Here's the drawing with two shaded views (mm, measured from the low corner). I have some questions. A direction names the side the tool comes from. Coordinates: 2 decimals unless noted, no trailing zeros. Loops run counter-clockwise (first coordinate to the right, second up) from the corner with the lowest first, then second, coordinate; pieces in that order, holes last.
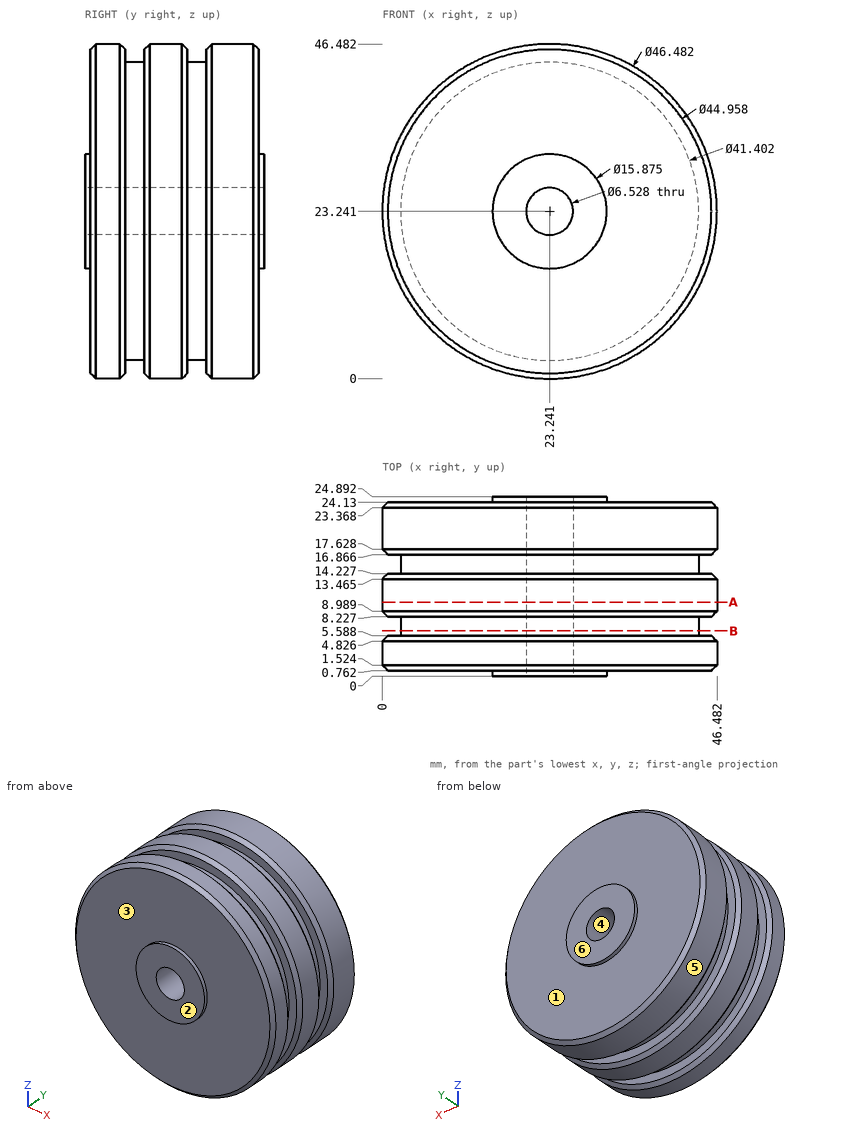
Q1. We'd pull the mould along Z, two halves only. Please class the marked faces 4, 5 and 6: pulls with the +Z half, pulls with the -Z half, needs draft (parallel to the pull), parting line crosses it, or undercut.
Q2. Suppose I cut it at B-B on y = 6.25. Write out the boundary of the cut face in (x, z).
Q3. For the marked faces 1, 2 and 3, which set-ups out of +Z, -Z, +X, -X, +Y, -Y let a thin tool reach every point of the face, with its end or its side?
Q4. Suppose I cut it at A-A on y = 10.25. Write out the boundary of the cut face in (x, z).
Q5. Please list where these lines run through material, in increasing order: probe 1 along Y at (x, z) = (18.5, 44) (1 decimal); probe 2 along Y at (x, z) = (33.5, 3) (1 decimal); probe 3 along Y at (x, z) = (14, 24.5).
Q6. Will these pins go through, and if not, where does the flat tip stop? P1, Ø4, axis at x = 8.5, z = 10.5, coming from the +Y side; P2, Ø6, axis at x = 39, y = 12, coming from the -Z side (1 decimal); P3, Ø10, axis at y = 7.5, z = 33.5, coming from the -X side.
Check values:
1. face 4: undercut
1. face 5: parting line crosses it
1. face 6: needs draft
2. outline: circle Ø41.4 at (23.24, 23.24); hole circle Ø6.53 at (23.24, 23.24)
3. face 1: +Y
3. face 2: +Z, -Z, +X, -X, -Y
3. face 3: -Y
4. outline: circle Ø46.48 at (23.24, 23.24); hole circle Ø6.53 at (23.24, 23.24)
5. probe 1: y = 0.8 to 5.6, 8.2 to 14.2, 16.9 to 24.1
5. probe 2: y = 1 to 5.4, 8.4 to 14, 17.1 to 23.9
5. probe 3: y = 0.76 to 24.13
6. P1: stops at y = 24.13
6. P2: stops at z = 3.8
6. P3: stops at x = 0.66
